Source: CAD feature listing. Evaluate the final solid. Frame: model axes, mm. A direction names the side the tool comes from. Give positions to 0.01 mm unless a question says otherwise; leave off trailing zeros. Loops run counter-clockwise (first coordinate to the right, second up) from the corner with the lowest first, then second, coordinate; pieces in that order, holes last.
from build123d import *

# Parameters (mm, degrees)
F0_R     = 17.145
F0_R_2   = 9.0724925833
F1_DEPTH = 88.9
F2_DEPTH = 25.4
F4_DEPTH = 88.901
F5_R     = 0.508
F7_DEPTH = 50.8


with BuildPart() as f1:
    # F0 (on Front) → F1 (new body)
    with BuildSketch(Plane.XZ):
        Circle(F0_R)
        Circle(F0_R_2, mode=Mode.SUBTRACT)
        Circle(F0_R_2)
    extrude(amount=F1_DEPTH)

    # F0 (on Front) → F2 (cut)
    with BuildSketch(Plane.XZ):
        Circle(F0_R_2)
    extrude(amount=F2_DEPTH, mode=Mode.SUBTRACT)

    # F3 (on face) → F4 (cut, through all)
    with BuildSketch(Plane.XZ.offset(88.9)):
        with BuildLine():
            ThreePointArc((-5.715, 14.5918745599), (0, 15.621), (5.715, 14.5918745599))
            Line((5.715, 14.5918745599), (5.715, 16.1644610179))
            ThreePointArc((5.715, 16.1644610179), (2.8992534253, 16.8980873053), (0, 17.145))
            ThreePointArc((0, 17.145), (-2.8992534253, 16.8980873053), (-5.715, 16.1644610179))
            Line((-5.715, 16.1644610179), (-5.715, 14.5918745599))
        make_face()
    extrude(amount=-F4_DEPTH, mode=Mode.SUBTRACT)

    # F5
    f5_edges = [f1.edges().sort_by_distance(p)[0] for p in [
        (-5.715, -44.45, 16.164461),
        (5.715, -44.45, 16.164461),
        (-5.715, -44.45, 14.591875),
        (5.715, -44.45, 14.591875),
    ]]
    fillet(f5_edges, radius=F5_R)

    # F6 (on face) → F7 (cut)
    with BuildSketch(Plane.XZ.offset(88.9)):
        with BuildLine():
            ThreePointArc((-3.0928797021, 8.7823797249), (-4.8083158044, 8.4599845105), (-6.5495779578, 8.5810869809))
            ThreePointArc((-6.5495779578, 8.5810869809), (0, -10.7950000092), (6.5495779578, 8.5810869809))
            ThreePointArc((6.5495779578, 8.5810869809), (4.8083158044, 8.4599845105), (3.0928797021, 8.7823797249))
            ThreePointArc((3.0928797021, 8.7823797249), (0, 9.2710000092), (-3.0928797021, 8.7823797249))
        make_face()
    extrude(amount=-F7_DEPTH, mode=Mode.SUBTRACT)


solid = f1.part
1) Cut plane A-A (y = -50). Return loops of the section in (x, z) (3 decimals), and give its area (3 significant figures).
Checks:
outline: (-6.413, 15.9) arc R17.145 ccw (long way) to (6.413, 15.9) arc R0.508 ccw to (5.715, 15.429) - (5.715, 15.306) arc R0.508 cw to (5.05, 14.823) arc R16.383 ccw to (-5.05, 14.823) arc R0.508 cw to (-5.715, 15.306) - (-5.715, 15.429) arc R0.508 ccw to start; hole (-6.55, 8.581) arc R10.795 ccw (long way) to (6.55, 8.581) arc R6.858 cw to (3.093, 8.782) arc R10.033 ccw to (-3.093, 8.782) arc R6.858 cw to start
area: 557 mm2
2) Pull-direction query (X, two-part tool) for faces 1 (the cylindrical face through (4.83, -63.86, 8.46)), 2 (the flat face through (7, 0, 7)), 3 (the cylindrical face through (-0.662, -43.828, -17.132)), 4 (the cylindrical face through (-4.78, -63.86, 8.46)); classes: released by +X, released by -X, zero draft, split by the parting line, or undercut.
Checks:
face 1: undercut
face 2: zero draft
face 3: split by the parting line
face 4: undercut
3) Reachability of faces 5 (the cylindrical face through (-0.07, -45.07, 15.62)), 6 (the cylindrical face through (8.65, -12.52, 2.73)), 7 (the cylindrical face through (-0.38, -63.86, -10.79)) from +Z, -Z, +X, -X, +Y, -Y: full face, straight path, thin tool, end or side. Return the list, or none.
Checks:
face 5: +Z, +Y, -Y
face 6: +Y
face 7: -Y
4) Contact query for flat-ended pins moving along their axis: P1, Ø3, axis at y = -28.5, z = 4, coming from the +X side; P2, Ø1.5, axis at x = 12.5, y = -21, coming from the +Z side; P3, Ø10, axis at y = -49, z = -9, coming from the -X side. Output: stop coordinate, or through.
Checks:
P1: stops at x = 16.96
P2: stops at z = 12.49
P3: stops at x = -16.67
5) Cut plane B-B (x = 0). Return loops of the section in (y, z) (1 decimal).
Checks:
outline: (-88.9, -17.1) - (0, -17.1) - (0, -9.1) - (-25.4, -9.1) - (-25.4, 9.1) - (0, 9.1) - (0, 15.6) - (-88.9, 15.6) - (-88.9, 9.3) - (-38.1, 9.3) - (-38.1, -10.8) - (-88.9, -10.8) - close
6) Cut plane C-C (z = 0). Return loops of the section in (x, y) (1 decimal).
Checks:
outline: (-17.1, -88.9) - (-10.8, -88.9) - (-10.8, -38.1) - (10.8, -38.1) - (10.8, -88.9) - (17.1, -88.9) - (17.1, 0) - (9.1, 0) - (9.1, -25.4) - (-9.1, -25.4) - (-9.1, 0) - (-17.1, 0) - close
7) Ray query, probe 1 along X at (y, z) = (-55, 0) (3 decimals); probe 2 along Z at (x, y) = (0, -13.5) (1 decimal); probe 3 along Y at (x, z) = (0.5, 0). Return the intervals inside material, ascending.
Checks:
probe 1: x = -17.145 to -10.795, 10.795 to 17.145
probe 2: z = -17.1 to -9.1, 9.1 to 15.6
probe 3: y = -38.1 to -25.4
8) Cut plane D-D (z = 13). Return loops of the section in (x, y), and give its area (3 significant figures).
Checks:
outline: (-11.18, -88.9) - (11.18, -88.9) - (11.18, 0) - (-11.18, 0) - close
area: 1,990 mm2
